Can you work these out from the model? Positions are in its coordinate system, mm. A direction names the side the tool comes from. Give positions to 0.01 mm unless a question says otherwise; leave off trailing zeros. Loops run counter-clockwise (first coordinate to the right, second up) from the corner with the lowest first, then second, coordinate; pieces in that order, holes last. Notation, with made-up numbers: (13.5, -38) - (57.5, -38) arc R12 ccw to (57.5, -25) - close; hole circle Ø6 at (15, 40). An arc over 180 degrees is marked (long way). Answer as a JSON object with one key per item and string values. Group by question number.
Item 1: Suppose I cut it at A-A on y = 12.7. Count the separate pieces of the cut face and the enclosed holes in it, and give its area (3 significant figures).
Item 2: Will these pins go through, and if not, where does the flat tip stop? pin 1 (4.5 mm diameter, centred on x = -31.75, z = -12.7, fed in from -Y); pin 2 (6.5 mm diameter, centred on x = 9, y = 10.5, fed in from +Z).
Item 3: Which directions (+Z, -Z, +X, -X, +Y, -Y) give clear straight access to the entire face, cutting with the end or side of a thin tool? Please do faces 1 (the flat face through (1, 23.812, -25)), 2 (the flat face through (1, 13, -50.8)).
Item 4: Please list where these lines run through material, in increasing order: L1, parallel to X at y = 24, z = -12.5; L2, parallel to Z at x = -31.75, y = 24.4; L3, parallel to Z at x = 34.5, y = 16.
Item 5: Suppose I cut it at B-B on x = -12.7. Write out the boundary of the cut face in (y, z).
Item 6: Thinking about a two-plate mould opening in X: for faces 3 (the flat face through (1, 13, 0)), 4 (the cylindrical face through (33.585, 14.382, -49.995)), 5 (the cylindrical face through (-32.29, 0.8, -35.67)), which applies, pulls with the +X half, pulls with the -X half, needs draft (parallel to the pull), parting line crosses it, or undercut?
Item 7: Suppose I cut it at D-D on y = 17.5. Write out the boundary of the cut face in (x, z), and give its area (3 significant figures).
Item 8: Suppose I cut it at C-C on z = -38.1. Write out the boundary of the cut face in (x, y).
from build123d import *

# Parameters (mm, degrees)
SKETCH1_W           = 50.8
SKETCH1_H           = 25.4
BOSS_EXTRUDE1_DEPTH = 44.45
SHELL1_T            = -1.5875
SKETCH2_R           = 2.4892
CUT_EXTRUDE1_DEPTH  = 26.4
SKETCH3_R           = 2.4892
CUT_EXTRUDE2_DEPTH  = 51.8
SKETCH4_R           = 2.5527
CUT_EXTRUDE3_DEPTH  = 51.8
CUT_EXTRUDE4_REACH  = 52.8
SKETCH5_R           = 2.5527


with BuildPart() as part:
    # Sketch1 → Boss-Extrude1 (new body, symmetric)
    with BuildSketch(Plane(origin=(0, 0, 0), x_dir=(0, 0, -1), z_dir=(1, 0, 0))):
        with Locations((25.4, 12.7)):
            Rectangle(SKETCH1_W, SKETCH1_H)
    extrude(amount=BOSS_EXTRUDE1_DEPTH, both=True)

    # Shell1
    shell1_openings = [part.faces().sort_by_distance(p)[0] for p in [
        (44.45, 12.7, -25.4),
        (-44.45, 12.7, -25.4),
    ]]
    offset(amount=SHELL1_T, openings=shell1_openings, kind=Kind.INTERSECTION)

    # Sketch2 → Cut-Extrude1 (cut, through all)
    with BuildSketch(Plane(origin=(0, 25.4, 0), x_dir=(1, 0, 0), z_dir=(0, 1, 0))):
        with Locations((-31.75, 25.4)):
            Circle(SKETCH2_R)
        with Locations((-31.75, 12.7)):
            Circle(SKETCH2_R)
        with Locations((-31.75, 38.1)):
            Circle(SKETCH2_R)
    cut_extrude1 = extrude(amount=-CUT_EXTRUDE1_DEPTH, mode=Mode.SUBTRACT)

    # Sketch3 → Cut-Extrude2 (cut, through all)
    with BuildSketch(Plane.XY):
        with Locations((-31.75, 12.7)):
            Circle(SKETCH3_R)
    cut_extrude2 = extrude(amount=-CUT_EXTRUDE2_DEPTH, mode=Mode.SUBTRACT)

    # Mirror1: Cut-Extrude1, Cut-Extrude2 across plane
    add(cut_extrude1.mirror(Plane(origin=(0, 0, 0), x_dir=(0, 0, 1), z_dir=(1, 0, 0))), mode=Mode.SUBTRACT)
    add(cut_extrude2.mirror(Plane(origin=(0, 0, 0), x_dir=(0, 0, 1), z_dir=(1, 0, 0))), mode=Mode.SUBTRACT)

    # Sketch4 → Cut-Extrude3 (cut, through all)
    with BuildSketch(Plane.XY):
        with Locations((-12.7, 12.7)):
            Circle(SKETCH4_R)
    extrude(amount=-CUT_EXTRUDE3_DEPTH, mode=Mode.SUBTRACT)

    # Sketch5 → Cut-Extrude4 (cut, up to next)
    with BuildSketch(Plane.XY, mode=Mode.PRIVATE) as cut_extrude4_sk1:
        with Locations((-31.75, 12.7)):
            Circle(SKETCH5_R)
    cut_extrude4_tool1 = extrude(cut_extrude4_sk1.sketch, amount=-CUT_EXTRUDE4_REACH, mode=Mode.PRIVATE) & part.part
    add(cut_extrude4_tool1.solids().sort_by_distance((-31.75, 12.7, 0))[0], mode=Mode.SUBTRACT)


solid = part.part
Worked out:
{
 "1": {"separate pieces": "8", "enclosed holes": "0", "area": "234 mm2"},
 "2": {"pin 1": "passes through", "pin 2": "stops at z = 0"},
 "3": {"face 1": "+X, -X", "face 2": "-Z, +X, -X, +Y, -Y"},
 "4": {"L1": "x = -44.45 to -34.23, -29.27 to 29.27, 34.23 to 44.45", "L2": "z = -50.8 to -40.59, -35.61 to -27.89, -22.91 to -15.19, -10.21 to 0", "L3": "z = -50.8 to -49.21, -1.59 to 0"},
 "5": {"outline": "(0, -50.8) - (10.15, -50.8) - (10.15, -49.21) - (1.59, -49.21) - (1.59, -1.59) - (10.15, -1.59) - (10.15, 0) - (0, 0) - close; (15.25, -50.8) - (25.4, -50.8) - (25.4, 0) - (15.25, 0) - (15.25, -1.59) - (23.81, -1.59) - (23.81, -49.21) - (15.25, -49.21) - close"},
 "6": {"face 3": "needs draft", "face 4": "undercut", "face 5": "undercut"},
 "7": {"outline": "(-44.45, -50.8) - (44.45, -50.8) - (44.45, -49.21) - (-44.45, -49.21) - close; (-44.45, -1.59) - (44.45, -1.59) - (44.45, 0) - (-44.45, 0) - close", "area": "282 mm2"},
 "8": {"outline": "(-44.45, 0) - (-34.24, 0) - (-34.24, 1.59) - (-44.45, 1.59) - close; (-44.45, 23.81) - (-34.24, 23.81) - (-34.24, 25.4) - (-44.45, 25.4) - close; (-29.26, 0) - (29.26, 0) - (29.26, 1.59) - (-29.26, 1.59) - close; (-29.26, 23.81) - (29.26, 23.81) - (29.26, 25.4) - (-29.26, 25.4) - close; (34.24, 0) - (44.45, 0) - (44.45, 1.59) - (34.24, 1.59) - close; (34.24, 23.81) - (44.45, 23.81) - (44.45, 25.4) - (34.24, 25.4) - close"}
}
